Part model, mm, in its own coordinate system. Round coordinates to 2 decimals unless told otherwise and drop trailing zeros. Write each loop counter-clockwise with the first axis right and the second up, starting at its lowest first coordinate (ties: lowest second). Pieces come first, ordered by that corner, then holes. Notation, with made-up numbers: M -12,31 L 2,31 A26 cw 2,46 Z; hole C 62,66.5 d1. An arc over 180 degrees is marked long. Answer as a JSON object with one key per item and string values. Group by question number.
1. Drill centre lines: line 1 (Z direction, x = -0.4, y = -0.2); line 2 (X direction, y = -0.1, z = 2.2); line 3 (Z direction, x = 0.45, y = -1.05). Where is each one in solid material? Low to high. Write a range as from..to.
2. Band-saw the part on C-C, the plane x = -0.65. Write the cut outline in (y, z), plus the area to 3 significant figures.
3. Band-saw the part on D-D, the plane x = -0.05. Write the cut outline in (y, z), plus the area to 3 significant figures.
4. Band-saw the part on A-A, the plane z = 0. Write the cut outline in (x, y).
5. Drop flat-ended pins along their axis: pin 1 (1 mm diameter, centred on x = 1.5, z = 1, fed in from +Y); pin 2 (1 mm diameter, centred on x = 0, z = 0.5, fed in from -Y). Give the stop position or say it passes through.
6. Two-plate mould, pull along Z, no slides. Class faces 1 (the face through (1.471, 0.338, -2.578)), 2 (the face through (2, 0, 2)), 3 (the face through (-0.03, 1.5, -0.07)): +Z half, -Z half, draft (parallel to the pull), parting line (faces both ways), or undercut.
from build123d import *

# Parameters (mm, degrees)
CHAMFER1_SIZE = 0.08


with BuildPart() as part:
    # Sketch1 → Revolve1 (revolve)
    with BuildSketch(Plane.XY):
        with BuildLine():
            Line((-2, -1.5), (-2, -2.6))
            Line((-2, -2.6), (-1.00871205, -2.6))
            ThreePointArc((-1.00871205, -2.6), (0, -2.05), (1.00871205, -2.6))
            Line((1.00871205, -2.6), (2, -2.6))
            Line((2, -2.6), (2, -1.5))
            Line((2, -1.5), (-2, -1.5))
        make_face()
    revolve(axis=Axis((-6.429017492, 0, 0), (1, 0, 0)))

    # Chamfer1
    chamfer1_edges = [part.edges().sort_by_distance(p)[0] for p in [
        (-2, 1.5, 0),
        (-2, 2.6, 0),
        (2, 2.6, 0),
        (2, 1.5, 0),
    ]]
    chamfer(chamfer1_edges, length=CHAMFER1_SIZE)


solid = part.part
Worked answers:
{
 "1": {"line 1": "z = -2.11..-1.49, 1.49..2.11", "line 2": "x = -2..-0.59, 0.59..2", "line 3": "z = -1.86..-1.07, 1.07..1.86"},
 "2": {"outline": "C 0,0 d4.48; hole C 0,0 d3", "area": "8.71 mm^2"},
 "3": {"outline": "C 0,0 d4.1; hole C 0,0 d3", "area": "6.15 mm^2"},
 "4": {"outline": "M -2,-2.52 L -1.92,-2.6 L -1.01,-2.6 A1.2 cw 1.01,-2.6 L 1.92,-2.6 L 2,-2.52 L 2,-1.58 L 1.92,-1.5 L -1.92,-1.5 L -2,-1.58 Z; M -2,1.58 L -1.92,1.5 L 1.92,1.5 L 2,1.58 L 2,2.52 L 1.92,2.6 L 1.01,2.6 A1.2 cw -1.01,2.6 L -1.92,2.6 L -2,2.52 Z"},
 "5": {"pin 1": "stops at y = 2.55", "pin 2": "stops at y = -2.12"},
 "6": {"face 1": "parting line", "face 2": "draft", "face 3": "undercut"}
}
